from build123d import *

# Parameters (mm, degrees)
BOSS_EXTRUDE1_DEPTH      = 0.8
SKETCH7_R                = 4
BOSS_EXTRUDE2_DEPTH      = 0.8
FILLET1_R                = 3
M2_CLEARANCE_HOLE1_D     = 2.4
M2_CLEARANCE_HOLE1_DEPTH = 30.5


with BuildPart() as part:
    # Sketch3 → Boss-Extrude1 (new body)
    with BuildSketch(Plane.XY):
        with BuildLine():
            Line((-40.732233047, 1.767766953), (-33.964466094, -5))
            Line((-33.964466094, -5), (33.964466094, -5))
            Line((33.964466094, -5), (40.732233047, 1.767766953))
            ThreePointArc((40.732233047, 1.767766953), (44.267766953, 1.767766953), (44.267766953, -1.767766953))
            Line((44.267766953, -1.767766953), (36.035533906, -10))
            Line((36.035533906, -10), (-36.035533906, -10))
            Line((-36.035533906, -10), (-44.267766953, -1.767766953))
            ThreePointArc((-44.267766953, -1.767766953), (-44.267766953, 1.767766953), (-40.732233047, 1.767766953))
        make_face()
    extrude(amount=BOSS_EXTRUDE1_DEPTH)

    # Sketch7 → Boss-Extrude2 (add)
    with BuildSketch(Plane.XY.offset(0.8)):
        with Locations((-42.5, 0)):
            Circle(SKETCH7_R)
        with Locations((42.5, 0)):
            Circle(SKETCH7_R)
    extrude(amount=-BOSS_EXTRUDE2_DEPTH)

    # Fillet1
    fillet1_edges = [part.edges().sort_by_distance(p)[0] for p in [
        (-33.964466094, -5, 0.4),
        (33.964466094, -5, 0.4),
        (-42.059826736, -3.97570717, 0.4),
        (-38.52429283, -0.440173264, 0.4),
        (42.059826736, -3.97570717, 0.4),
        (38.52429283, -0.440173264, 0.4),
    ]]
    fillet(fillet1_edges, radius=FILLET1_R)

    # M2 Clearance Hole1
    with Locations(Plane.XY.offset(0.8)):
        with Locations((-42.5, 0), (42.5, 0)):
            Hole(M2_CLEARANCE_HOLE1_D / 2, depth=M2_CLEARANCE_HOLE1_DEPTH)


solid = part.part
Can you work these out from the model? Positions are in its coordinate system, mm. A direction names the side the tool comes from. Coordinates: 2 decimals unless noted, no trailing zeros. Loops run counter-clockwise (first coordinate to the right, second up) from the corner with the lowest first, then second, coordinate; pieces in that order, holes last. Notation, with made-up numbers: (61, 13.5) - (77, 13.5) arc R20 ccw to (77, 35.5) - close; hole circle Ø2 at (62, 42.25). An arc over 180 degrees is marked (long way). Answer as a JSON object with one key per item and string values. Group by question number.
Item 1: If I drill on L1, parallel to X at y = -1, z = 0.65; L2, parallel to X at y = -0.5, z = 0.6; L3, parallel to Y at x = -10.5, z = 0.55, over which ranges is the centre line in solid material (lowest first)? Write a range as from..to.
Item 2: For pin 1 (3 mm diameter, centred on x = 42.5, y = 0, fed in from -Z), with a flat end and sliding along its axis, tell me the tip position at first contact or that it passes through.
Item 3: If we section it at B-B (y = -2.5): List the corners of the cut face in (x, z) for me, plus the area to 3 significant figures.
Item 4: If we mould it in two halves opening along X, with no side actions, what happens to faces 3 (the face through (-43.61, -0.46, 0.39)), 4 (the face through (-36.277, -2.688, 0.394)), 5 (the face through (-1, -6, 0.8)), 6 (the face through (38.657, -7.379, 0.394))? For each: released by +X, released by -X, zero draft, split by the parting line, or undercut.
Item 5: If we section it at C-C (x = 10.5): List the corners of the cut face in (y, z) for me.
Item 6: If we section it at A-A (z = 0.6): List the corners of the cut face in (x, y) for me, plus the area to 3 significant figures.
Item 7: On a 3-axis mill with a long thin cutter (end or side, diameter ignored), from which of +Z, -Z, +X, -X, +Y, -Y can I reach the whole of each face in a straight line? I mean faces 1 (the face through (-38.585, -7.451, 0.394)), 2 (the face through (36.237, -2.727, 0.394)). Say none if no direction works.
Item 8: If we section it at D-D (y = 2): List the corners of the cut face in (x, z) for me.
Returned:
{
 "1": {"L1": "x = -46.37..-43.16, -41.84..-37.93, 37.93..41.84, 43.16..46.37", "L2": "x = -46.47..-43.59, -41.41..-38.24, 38.24..41.41, 43.59..46.47", "L3": "y = -10..-5"},
 "2": {"pin 1": "stops at z = 0"},
 "3": {"outline": "(-45.62, 0) - (-36.46, 0) - (-36.46, 0.8) - (-45.62, 0.8) - close; (36.46, 0) - (45.62, 0) - (45.62, 0.8) - (36.46, 0.8) - close", "area": "14.7 mm²"},
 "4": {"face 3": "undercut", "face 4": "undercut", "face 5": "zero draft", "face 6": "released by +X"},
 "5": {"outline": "(-10, 0) - (-5, 0) - (-5, 0.8) - (-10, 0.8) - close"},
 "6": {"outline": "(-42.97, -3.97) arc R3 cw to (-41.21, -4.83) - (-36.04, -10) - (36.04, -10) - (41.21, -4.83) arc R3 cw to (42.97, -3.97) arc R4 ccw (long way) to (38.53, 0.47) arc R3 cw to (37.67, -1.29) - (34.84, -4.12) arc R3 cw to (32.72, -5) - (-32.72, -5) arc R3 cw to (-34.84, -4.12) - (-37.67, -1.29) arc R3 cw to (-38.53, 0.47) arc R4 ccw (long way) to start; hole circle Ø2.4 at (-42.5, 0); hole circle Ø2.4 at (42.5, 0)", "area": "511 mm²"},
 "7": {"face 1": "+Z, -Z, -X, -Y", "face 2": "+Z, -Z, +Y"},
 "8": {"outline": "(-45.96, 0) - (-39.04, 0) - (-39.04, 0.8) - (-45.96, 0.8) - close; (39.04, 0) - (45.96, 0) - (45.96, 0.8) - (39.04, 0.8) - close"}
}
